from build123d import *

# Parameters (mm, degrees)
BOX_W           = 6.5
BOX_H           = 14
BOX_DEPTH       = 14
SKETCH_W        = 3.5
SKETCH_H        = 1
POCKET_DEPTH    = 14
SKETCH001_W     = 3.5
SKETCH001_H     = 1.2
POCKET001_DEPTH = 14
CHAMFER_SIZE    = 1
CHAMFER001_SIZE = 1
CHAMFER002_SIZE = 1
CHAMFER003_SIZE = 1


with BuildPart() as part:
    # Box → Box (new body)
    with BuildSketch(Plane.XY):
        with Locations((3.25, 7)):
            Rectangle(BOX_W, BOX_H)
    extrude(amount=BOX_DEPTH)

    # Sketch → Pocket (cut)
    with BuildSketch(Plane.XY.offset(14)):
        with Locations((3.25, 13.5)):
            Rectangle(SKETCH_W, SKETCH_H)
        with Locations((3.25, 0.5)):
            Rectangle(SKETCH_W, SKETCH_H)
    extrude(amount=-POCKET_DEPTH, mode=Mode.SUBTRACT)

    # Sketch001 → Pocket001 (cut)
    with BuildSketch(Plane.XZ.offset(-1)):
        with Locations((3.25, 13.4)):
            Rectangle(SKETCH001_W, SKETCH001_H)
        with Locations((3.25, 0.6)):
            Rectangle(SKETCH001_W, SKETCH001_H)
    extrude(amount=-POCKET001_DEPTH, mode=Mode.SUBTRACT)

    # Chamfer
    chamfer_edges = [part.edges().sort_by_distance(p)[0] for p in [
        (3.25, 1, 12.8),
    ]]
    chamfer(chamfer_edges, length=CHAMFER_SIZE)

    # Chamfer001
    chamfer001_edges = [part.edges().sort_by_distance(p)[0] for p in [
        (3.25, 1, 1.2),
    ]]
    chamfer(chamfer001_edges, length=CHAMFER001_SIZE)

    # Chamfer002
    chamfer002_edges = [part.edges().sort_by_distance(p)[0] for p in [
        (3.25, 13, 12.8),
    ]]
    chamfer(chamfer002_edges, length=CHAMFER002_SIZE)

    # Chamfer003
    chamfer003_edges = [part.edges().sort_by_distance(p)[0] for p in [
        (3.25, 13, 1.2),
    ]]
    chamfer(chamfer003_edges, length=CHAMFER003_SIZE)


solid = part.part
Input: part model. Units: mm. Frame: model coordinates. A direction names the side the tool comes from. Coordinates: 2 decimals unless noted, no trailing zeros. Loops run counter-clockwise (first coordinate to the right, second up) from the corner with the lowest first, then second, coordinate; pieces in that order, holes last. Notation, with made-up numbers: (-23.5, 84) - (3.5, 84) arc R16 cw to (3.5, 93) - close; hole circle Ø8 at (14.5, 57). An arc over 180 degrees is marked (long way). Answer in a Markdown table with one row per item. Add a question column.
Item 1: Section query C-C on y = 12.25. Return the cut outline in (x, z).
Item 2: Access query for faces 1 (the flat face through (3, 7, 1.2)), 2 (the flat face through (5, 0.7, 7.1)), 3 (the flat face through (3.2, 12.5, 1.7)), 4 (the flat face through (3, 13, 7)). Directions: +Z, -Z, +X, -X, +Y, -Y. A direction counts if a zero-diameter tool reaches every point of the face in a straight line with its end or side. Return the directions, or none.
Item 3: Section query B-B on x = 4. Return the cut outline in (y, z), then the cut area to 3 significant figures.
Item 4: Section query A-A on z = 7.5. Return the cut outline in (x, y), then the cut area to 3 significant figures.
Item 5: Mould query, pull axis X, two halves, no side actions, for faces 5 (the flat face through (6.5, 7, 7)), 6 (the flat face through (3, 7, 12.8)), 7 (the flat face through (0, 7, 7)), 8 (the flat face through (1, 0, 7)). Classes: released by +X, released by -X, zero draft, split by the parting line, or undercut.
Item 6: Line query: line 1 along X through (y, z) = (11.75, 13); line 2 along Z through (x, y) = (2.25, 8); line 3 along Y through (x, z) = (2.5, 11). Output: solid intervals per line, ascending. Write a range as [from, to].
Item 7: Contact query for flat-ended pins moving along their axis: P1, Ø3, axis at x = 5, z = 2, coming from the -Y side; P2, Ø1.8, axis at x = 3, y = 8.5, coming from the +Z side; P3, Ø1, axis at x = 3.5, y = 7.5, coming from the -Z side. Output: stop coordinate, or through.
Recorded:
| question | item | result |
|---|---|---|
| 1 | outline | (0, 0) - (1.5, 0) - (1.5, 1.45) - (5, 1.45) - (5, 0) - (6.5, 0) - (6.5, 14) - (5, 14) - (5, 12.55) - (1.5, 12.55) - (1.5, 14) - (0, 14) - close |
| 2 | face 1 | -Z, +Y, -Y |
| 2 | face 2 | none |
| 2 | face 3 | -Z, +Y |
| 2 | face 4 | +Z, -Z, +Y |
| 3 | outline | (1, 2.2) - (2, 1.2) - (12, 1.2) - (13, 2.2) - (13, 11.8) - (12, 12.8) - (2, 12.8) - (1, 11.8) - close |
| 3 | area | 137 mm^2 |
| 4 | outline | (0, 0) - (1.5, 0) - (1.5, 1) - (5, 1) - (5, 0) - (6.5, 0) - (6.5, 14) - (5, 14) - (5, 13) - (1.5, 13) - (1.5, 14) - (0, 14) - close |
| 4 | area | 84.0 mm^2 |
| 5 | face 5 | released by +X |
| 5 | face 6 | undercut |
| 5 | face 7 | released by -X |
| 5 | face 8 | zero draft |
| 6 | line 1 | [0, 1.5], [5, 6.5] |
| 6 | line 2 | [1.2, 12.8] |
| 6 | line 3 | [1, 13] |
| 7 | P1 | y = 0 |
| 7 | P2 | z = 12.8 |
| 7 | P3 | z = 1.2 |
